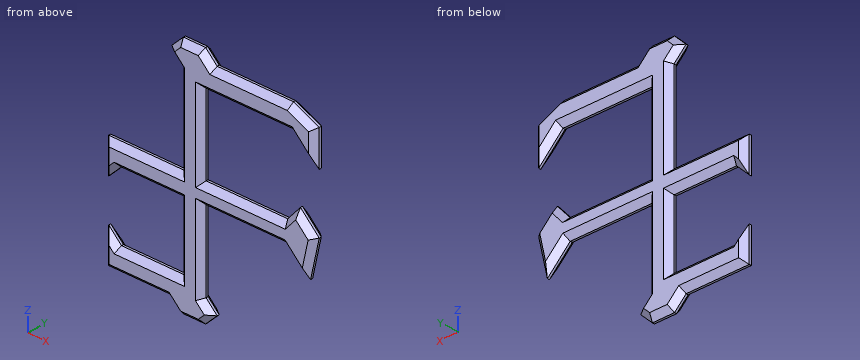
```python
from build123d import *

# Parameters (mm, degrees)
F1_DEPTH = 3.81
F2_SIZE  = 1.5875
F3_SCALE = 0.75


with BuildPart() as f1:
    # F0 (on Front) → F1 (new body)
    with BuildSketch(Plane.XZ):
        Polygon((-6.6455395231, 29.4341069916), (-3.175, 25.9635674685), (-3.175, 0.1128360473), (-24.7444733058, 0.1128360473), (-24.7444733058, -9.883693457), (-21.0979438016, -6.2371639527), (-3.175, -6.2371639527), (-3.175, -25.5762760587), (-21.0979438016, -25.5762760587), (-24.7444733058, -21.9297465545), (-24.7444733058, -31.9262760587), (-22.1278171024, -31.9262760587), (-6.6455395231, -31.9262760587), (-3.3227697615, -35.2490458202), (3.0272302385, -35.2490458202), (6.35, -31.9262760587), (3.175, -28.7512760587), (3.175, -5.8234985377), (26.6026397626, -5.8234985377), (33.1378690898, -12.3587278649), (35.6206595898, -1.1474714229), (30.2332143891, 4.2399737777), (26.6026397626, 0), (3.175, 0), (3.175, 22.7885674685), (28.6609344184, 22.7885674685), (35.6206595898, 15.7537590712), (35.6206595898, 26.0716768982), (28.2596744327, 29.4341069916), (6.35, 29.4341069916), (3.0272302385, 32.7568767531), (-3.3227697615, 32.7568767531), align=None)
    extrude(amount=F1_DEPTH)

    # F2
    f2_edges = [f1.edges().sort_by_distance(p)[0] for p in [
        (17.304837, -3.81, 29.434107),
        (4.688615, -3.81, 31.095492),
        (-0.14777, -3.81, 32.756877),
        (-4.984155, -3.81, 31.095492),
        (-4.91027, -3.81, 27.698837),
        (-3.175, -3.81, 13.038202),
        (-13.959737, -3.81, 0.112836),
        (-24.744473, -3.81, -4.885429),
        (-22.921209, -3.81, -8.060429),
        (-12.136472, -3.81, -6.237164),
        (-3.175, -3.81, -15.90672),
        (-12.136472, -3.81, -25.576276),
        (-22.921209, -3.81, -23.753011),
        (-24.744473, -3.81, -26.928011),
        (-15.695006, -3.81, -31.926276),
        (-4.984155, -3.81, -33.587661),
        (-0.14777, -3.81, -35.249046),
        (4.688615, -3.81, -33.587661),
        (4.7625, -3.81, -30.338776),
        (3.175, -3.81, -17.287387),
        (14.88882, -3.81, -5.823499),
        (29.870254, -3.81, -9.091113),
        (34.379264, -3.81, -6.7531),
        (32.926937, -3.81, 1.546251),
        (28.417927, -3.81, 2.119987),
        (14.88882, -3.81, 0),
        (3.175, -3.81, 11.394284),
        (15.917967, -3.81, 22.788567),
        (32.140797, -3.81, 19.271163),
        (35.62066, -3.81, 20.912718),
        (31.940167, -3.81, 27.752892),
        (17.304837, 0, 29.434107),
        (4.688615, 0, 31.095492),
        (-0.14777, 0, 32.756877),
        (-4.984155, 0, 31.095492),
        (-4.91027, 0, 27.698837),
        (-3.175, 0, 13.038202),
        (-13.959737, 0, 0.112836),
        (-24.744473, 0, -4.885429),
        (-22.921209, 0, -8.060429),
        (-12.136472, 0, -6.237164),
        (-3.175, 0, -15.90672),
        (-12.136472, 0, -25.576276),
        (-22.921209, 0, -23.753011),
        (-24.744473, 0, -26.928011),
        (-15.695006, 0, -31.926276),
        (-4.984155, 0, -33.587661),
        (-0.14777, 0, -35.249046),
        (4.688615, 0, -33.587661),
        (4.7625, 0, -30.338776),
        (3.175, 0, -17.287387),
        (14.88882, 0, -5.823499),
        (29.870254, 0, -9.091113),
        (34.379264, 0, -6.7531),
        (32.926937, 0, 1.546251),
        (28.417927, 0, 2.119987),
        (14.88882, 0, 0),
        (3.175, 0, 11.394284),
        (15.917967, 0, 22.788567),
        (32.140797, 0, 19.271163),
        (35.62066, 0, 20.912718),
        (31.940167, 0, 27.752892),
    ]]
    chamfer(f2_edges, length=F2_SIZE)


with BuildPart() as f1_1:
    # F3: moved
    add(f1.part.scale(F3_SCALE))


solid = f1_1.part
```
Read the model definition and answer for the solid it produces. Units are mm, in the model's axes. Round coordinates to 2 decimals unless told otherwise and drop trailing zeros. Write each loop counter-clockwise with the first axis right and the second up, starting at its lowest first coordinate (ties: lowest second). Pieces come first, ordered by that corner, then holes. Notation, with made-up numbers: (67, 17.5) - (76, 17.5) arc R32 ccw to (76, 53.5) - close; hole circle Ø2 at (67, 22). An arc over 180 degrees is marked (long way). Use CSV: the item, a comma, the result in double quotes.
Q1. Find section B-B, the plane z = -14.5. Write down the section's boundary in (x, y).
Values:
outline,"(-2.38, -1.67) - (-1.19, -2.86) - (1.19, -2.86) - (2.38, -1.67) - (2.38, -1.19) - (1.19, 0) - (-1.19, 0) - (-2.38, -1.19) - close"
Q2. Each of these flat-tipped pins is pushed along its axis until it touches: pin 1 Ø12 at (x, z) = (2.5, 15.5) entering from -Y; pin 2 Ø0.5 at (x, y) = (-8.5, -1.5) entering from -Z; pin 3 Ø0.5 at (y, z) = (-1.5, -11.5) entering from -X. Where does it stop, or does it pass through?
Values:
pin 1,"stops at y = -2.86"
pin 2,"stops at z = -23.94"
pin 3,"stops at x = -2.38"
Q3. Straight lines are drawn through the part: line 1 along X through (y, z) = (-2.45, -4); line 2 along Z through (x, y) = (-3, -1.2); line 3 along Z through (x, y) = (-8, -1.4). For each, find the intervals that lie inside material, in ascending order.
Values:
line 1,"x = -17.78 to -16.25, -1.6 to 1.6, 20.69 to 25.22"
line 2,"z = -25.93 to -19.18, -4.68 to 0.08, 20.09 to 24.06"
line 3,"z = -23.94 to -19.18, -4.68 to 0.08"
Q4. Find section C-C, the plane x = 0.5. Write down the section's boundary in (y, z), then the cut area to 3 significant figures.
Values:
outline,"(-2.86, -25.25) - (-1.67, -26.44) - (-1.19, -26.44) - (0, -25.25) - (0, 23.38) - (-1.19, 24.57) - (-1.67, 24.57) - (-2.86, 23.38) - close"
area,"143 mm²"
Q5. Find section A-A, the plane x = 16. Write down the section's boundary in (y, z), then the cut area to 3 significant figures.
Values:
outline,"(-2.86, -3.18) - (-1.67, -4.37) - (-1.19, -4.37) - (0, -3.18) - (0, -1.19) - (-1.19, 0) - (-1.67, 0) - (-2.86, -1.19) - close; (-2.86, 18.28) - (-1.67, 17.09) - (-1.19, 17.09) - (0, 18.28) - (0, 20.88) - (-1.19, 22.08) - (-1.67, 22.08) - (-2.86, 20.88) - close"
area,"21.1 mm²"
